from build123d import *


with BuildPart() as part:
    # Torch_Plug Sketch → Torch_Plug (revolve)
    with BuildSketch(Plane.XY, mode=Mode.PRIVATE) as torch_plug_sk:
        Polygon((-33.4, 0), (-33.4, 4.5), (-42, 4.5), (-42, 8), (-50, 8), (-50, 7), (-76, 7), (-76, 0), align=None)
    revolve(torch_plug_sk.sketch.rotate(Axis((-300, 0, 0), (1, 0, 0)), 90), axis=Axis((-300, 0, 0), (1, 0, 0)))


solid = part.part
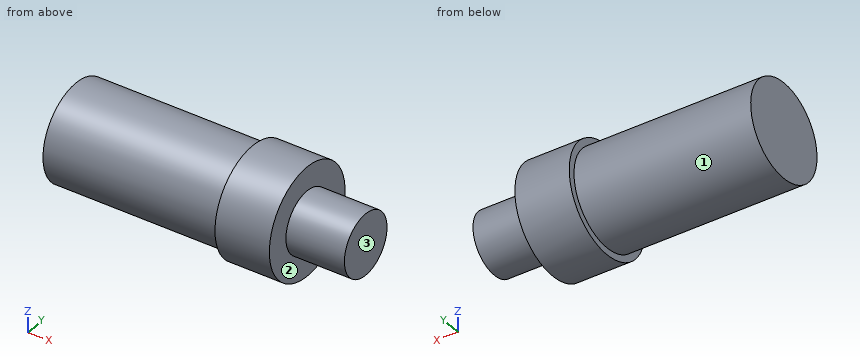
Input: part model. Units: mm. Frame: model coordinates. Face numbers are marked on the shaded views. A direction names the side the tool comes from. Coordinates: 2 decimals unless noted, no trailing zeros. Order: outer loops, then holes, each group sorted by start corner. A loop starts at its lowest first (then second) coordinate and runs counter-clockwise, first axis right, second up. Notation, with made-up numbers: M 34.5,-20 L 51.5,-20 A35 cw 51.5,18 Z; hole C 67,28.25 d8. An arc over 180 degrees is marked long. Answer as CSV lines item,"result".
1. Material intervals for line 1 (X direction, y = 0.75, z = -6.5); line 2 (X direction, y = 5, z = -5.5); line 3 (Z direction, x = -65, y = -0.5), sorted ascending. Write a range as from..to.
Reported:
line 1,"-76..-42"
line 2,"-50..-42"
line 3,"-6.98..6.98"
2. Access query for the marked faces 1, 2 and 3. Directions: +Z, -Z, +X, -X, +Y, -Y. A direction counts if a zero-diameter tool reaches every point of the face in a straight line with its end or side. Return the directions, or none.
Reported:
face 1,"-X"
face 2,"+X"
face 3,"+Z, -Z, +X, +Y, -Y"
3. First-contact query: P1, Ø5, axis at x = -53.5, y = 4, coming from the -Z side; P2, Ø6, axis at x = -56, z = -4.5, coming from the +Y side; P3, Ø1.5, axis at x = -65.5, y = -2, coming from the +Z side; P4, Ø4, axis at x = -42.5, y = 1.5, coming from the -Z side. Flat tips, straight axial feed; report the tip coordinate or a pass-through.
Reported:
P1,"z = -6.84"
P2,"y = 6.84"
P3,"z = 6.89"
P4,"z = -8"
4. Section A-A (z = 0). Return the cut outline in (x, y).
Reported:
outline,"M -76,-7 L -50,-7 L -50,-8 L -42,-8 L -42,-4.5 L -33.4,-4.5 L -33.4,4.5 L -42,4.5 L -42,8 L -50,8 L -50,7 L -76,7 Z"
5. Section C-C (x = -39.5). Return the cut outline in (y, z), then the cut area to 3 significant figures.
Reported:
outline,"C 0,0 d9"
area,"63.6 mm2"
6. Section D-D (z = 6.5). Return the cut outline in (x, y).
Reported:
outline,"M -76,-2.6 L -50,-2.6 L -50,-4.66 L -42,-4.66 L -42,4.66 L -50,4.66 L -50,2.6 L -76,2.6 Z"
